Geometry check sheet. Reference: the model listing, model coordinates, mm. Face numbers are marked on the shaded views. A direction names the side the tool comes from. Round coordinates to 2 decimals unless told otherwise and drop trailing zeros. Order: outer loops, then holes, each group sorted by start corner. A loop starts at its lowest first (then second) coordinate and runs counter-clockwise, first axis right, second up. Notation, with made-up numbers: M 2.5,-5 L 20.5,-5 A34 cw 20.5,27 Z; hole C 19,-20.75 d3. An arc over 180 degrees is marked long. Return JSON: item names as keys, results as strings. Group by question number.
```python
from build123d import *

# Parameters (mm, degrees)
F2_W     = 25.016323
F2_H     = 27.49747
F3_DEPTH = 25.4
F0_R     = 63.612596
F1_R     = 32.019182
F4_DEPTH = 25.4
F5_R     = 50.830077
F6_DEPTH = 25.4


with BuildPart() as f3:
    # F2 (on face) → F3 (new body)
    with BuildSketch(Plane.XZ):
        with Locations((0.191535, -0.859296)):
            Rectangle(F2_W, F2_H)
    extrude(amount=F3_DEPTH)

    # F0 (on Front) + F1 (on face) → F4 (join)
    with BuildSketch(Plane.XZ):
        Circle(F0_R)
    with BuildSketch(Plane.XZ):
        Circle(F1_R)
    extrude(amount=F4_DEPTH)

    # F5 (on face) → F6 (join)
    with BuildSketch(Plane.XZ.offset(25.4)):
        Circle(F5_R)
    extrude(amount=F6_DEPTH)


solid = f3.part
```
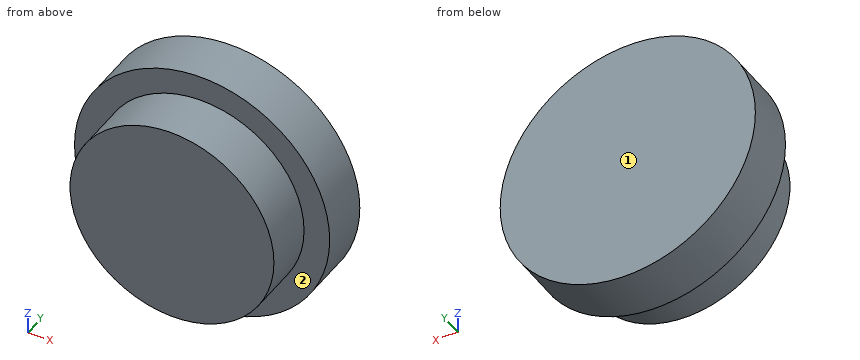
Q1. Section check D-D on y = -41. Record the cut outline in (x, z), plus the area to 3 significant figures.
Q2. Section check A-A on z = 0. Record the cut outline in (x, y).
Q3. Set-up check for the marked faces 1 and 2: record each of +Z, -Z, +X, -X, +Y, -Y from which the full face is reachable in a straight line by a thin tool's end or side.
Q4. Section check C-C on y = -6. Record the cut outline in (x, z).
Q5. Depth check by flat-ended pin: pin 1 Ø12 at (x, z) = (-31, -34) entering from +Y; pin 2 Ø3 at (x, y) = (8, -35) entering from +Z; pin 3 Ø8 at (y, z) = (-7, -33) entering from -X; pin 4 Ø5 at (y, z) = (-21.5, -32.5) entering from -X. Enter the tip coordinate at first touch or a pass-through.
Q6. Section check B-B on x = 0. Record the cut outline in (y, z), plus the area to 3 significant figures.
Q7. Material ranges on line 1 along Z through (x, y) = (1.5, -19); line 2 along Y through (x, z) = (2.5, -56.5), recorded low to high.
Geometry check:
{
 "1": {"outline": "C 0,0 d101.66", "area": "8,120 mm^2"},
 "2": {"outline": "M -63.61,-25.4 L -50.83,-25.4 L -50.83,-50.8 L 50.83,-50.8 L 50.83,-25.4 L 63.61,-25.4 L 63.61,0 L -63.61,0 Z"},
 "3": {"face 1": "+Z, -Z, +X, -X, +Y", "face 2": "-Y"},
 "4": {"outline": "C 0,0 d127.23"},
 "5": {"pin 1": "stops at y = 0", "pin 2": "stops at z = 50.41", "pin 3": "stops at x = -56.62", "pin 4": "stops at x = -56.09"},
 "6": {"outline": "M -50.8,-50.83 L -25.4,-50.83 L -25.4,-63.61 L 0,-63.61 L 0,63.61 L -25.4,63.61 L -25.4,50.83 L -50.8,50.83 Z", "area": "5,810 mm^2"},
 "7": {"line 1": "z = -63.59 to 63.59", "line 2": "y = -25.4 to 0"}
}
